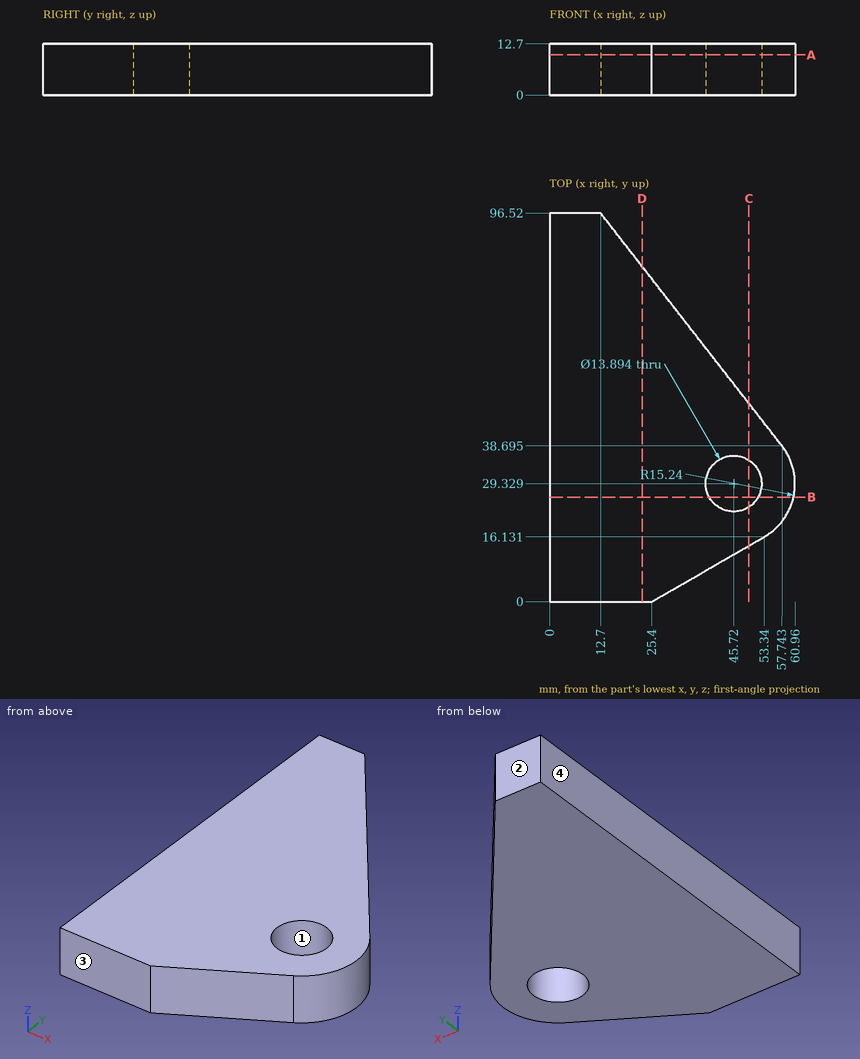
Check sheet for the drawn part. Datum: minimum x, y, z corner. Units: mm. Give positions to 0.01 mm unless a question says otherwise; leave off trailing zeros. Order: outer loops, then holes, each group sorted by start corner. A loop starts at its lowest first (then second) coordinate and runs counter-clockwise, first axis right, second up. Notation, with made-up numbers: (28, -1) - (42, -1) arc R3 ccw to (42, 3) - close; hole circle Ø1 at (11.25, 85). An arc over 180 degrees is marked (long way). Write item = value, one per line. Start each with the question number.
1) Scan lines: L1, parallel to Y at x = 45.72, z = 6.5 (1 decimal); L2, parallel to X at y = 26.5, z = 5.75 (1 decimal); L3, parallel to X at y = 60, z = 5.5. Record each from-to range of solid material in increasing order.
2) Section check D-D (x = 23). Enter the section's corners in (y, z), then the cut area to 3 significant figures.
3) Section check C-C (x = 49.5). Enter the section's corners in (y, z).
4) Section check A-A (z = 10). Enter the section's corners in (x, y) (1 decimal), then the cut area to 3 significant figures.
5) Gauge pin test, flat ends, axial feed: pin 1 Ø1.5 at (x, z) = (51, 2) entering from +Y (1 decimal); pin 2 Ø12.5 at (x, y) = (45.72, 29.33) entering from +Z; pin 3 Ø4 at (x, z) = (51, 10) entering from -Y (1 decimal). Record the tip position at first contact, or that the pin passes through.
6) Draft check along Y on the marked faces 1, 2, 3 and 4. Enter one of: released by +Y, released by -Y, zero draft, split by the parting line, or undercut.
7) Section check B-B (y = 26). Enter the section's corners in (x, z), then the cut area to 3 significant figures.
Geometry check:
q1.L1 = 11.7 to 22.4, 36.3 to 54.1
q1.L2 = 0 to 39.4, 52.1 to 60.7
q1.L3 = 0 to 41.15
q2.outline = (0, 0) - (83.3, 0) - (83.3, 12.7) - (0, 12.7) - close
q2.area = 1,060 mm2
q3.outline = (13.91, 0) - (23.5, 0) - (23.5, 12.7) - (13.91, 12.7) - close; (35.16, 0) - (49.28, 0) - (49.28, 12.7) - (35.16, 12.7) - close
q4.outline = (0, 0) - (25.4, 0) - (53.3, 16.1) arc R15.2 ccw to (57.7, 38.7) - (12.7, 96.5) - (0, 96.5) - close; hole circle Ø13.9 at (45.7, 29.3)
q4.area = 3,860 mm2
q5.pin_1 = 48.3
q5.pin_2 = through
q5.pin_3 = 13.6
q6.face_1 = undercut
q6.face_2 = released by +Y
q6.face_3 = released by -Y
q6.face_4 = zero draft
q7.outline = (0, 0) - (39.62, 0) - (39.62, 12.7) - (0, 12.7) - close; (51.82, 0) - (60.59, 0) - (60.59, 12.7) - (51.82, 12.7) - close
q7.area = 615 mm2
